Source: CAD feature listing. Evaluate the final solid. Frame: model axes, mm. Face numbers are marked on the shaded views. A direction names the side the tool comes from. Round coordinates to 2 decimals unless told otherwise and drop trailing zeros. Order: outer loops, then holes, each group sorted by start corner. A loop starts at its lowest first (then second) coordinate and runs counter-clockwise, first axis right, second up. Notation, with made-up numbers: M 73,-24 L 124,-24 A24 cw 124,9 Z; hole C -9.5,15.25 d11. An arc over 180 degrees is marked long. Use one line per item in the form item = value. Start each with the question number.
Q1. Reachability of the marked faces 1, 2, 3 and 4 from +Z, -Z, +X, -X, +Y, -Y: full face, straight path, thin tool, end or side. Return the list, or none.
Q2. Section C-C (y = -5). Return the cut outline in (x, z).
Q3. Section B-B (x = -6). Return the cut outline in (y, z), plus the area to 3 significant figures.
Q4. Pull-direction query (X, two-part tool) for the marked faces 5, 6, 7 and 8; classes: pulls with the +X half, pulls with the -X half, needs draft (parallel to the pull), parting line crosses it, or undercut.
Q5. Section D-D (y = -11). Return the cut outline in (x, z).
Q6. Section A-A (z = 4). Return the cut outline in (x, y), plus the area to 3 significant figures.
Q7. Material intervals for probe 1 along Z at (x, y) = (4, -3); probe 2 along Y at (x, z) = (-6, -2); probe 3 along X at (y, z) = (-1.25, 5.25), sorted ascending.
Q8. Contact query for flat-ended pins moving along their axis: pin 1 (2 mm diameter, centred on x = -2.5, y = -7.5, fed in from +Z); pin 2 (2 mm diameter, centred on x = 1, y = -2.5, fed in from -Z); pin 3 (3 mm diameter, centred on x = 8.5, y = -2.5, fed in from +Z); pin 4 (2.5 mm diameter, centred on x = -6, z = 4, fed in from -Y). Output: stop coordinate, or through.
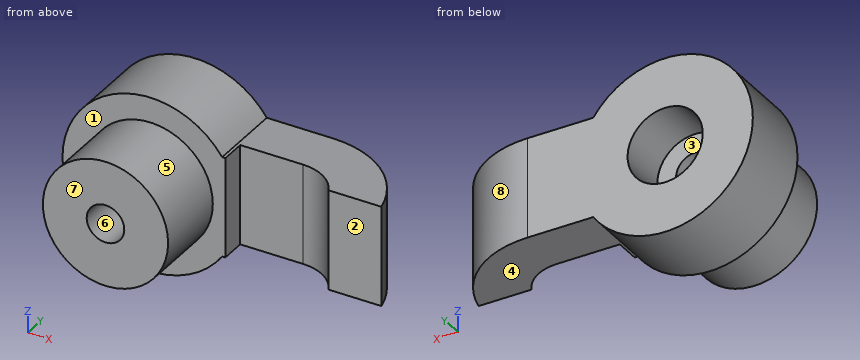
from build123d import *

# Parameters (mm, degrees)
EXTRUDE_1_DEPTH           = 8
EXTRUDE_2_DEPTH           = 6
SKETCH_5_R                = 5
EXTRUDE_3_DEPTH           = 6
HOLE_WIZARD_1_D           = 3
HOLE_WIZARD_1_DEPTH       = 30
HOLE_WIZARD_1_CBORE_D     = 6
HOLE_WIZARD_1_CBORE_DEPTH = 4


with BuildPart() as part:
    # 草图3 → 凸台-拉伸1 (new body)
    with BuildSketch(Plane.XY):
        with BuildLine():
            Line((0, 0), (5, 0))
            ThreePointArc((5, 0), (9.784396345, -1.68635165), (12.453978369, -6))
            Line((12.453978369, -6), (8.243547108, -6))
            ThreePointArc((8.243547108, -6), (6.905295111, -4.540192237), (5, -4))
            Line((5, -4), (0, -4))
            Line((0, -4), (0, 0))
        make_face()
    extrude(amount=EXTRUDE_1_DEPTH)

    # 草图4 → 凸台-拉伸2 (add)
    with BuildSketch(Plane(origin=(0, 0, 0), x_dir=(1, 0, 0), z_dir=(0, 1, 0))):
        with BuildLine():
            Line((-0.255437353, 0), (0, 0))
            Line((0, 0), (0, -8))
            Line((0, -8), (-0.255437353, -8))
            ThreePointArc((-0.255437353, -8), (-13, -4), (-0.255437353, 0))
        make_face()
    extrude(amount=-EXTRUDE_2_DEPTH)

    # 草图5 → 凸台-拉伸3 (add)
    with BuildSketch(Plane.XZ.offset(6)):
        with Locations((-6, 4)):
            Circle(SKETCH_5_R)
    extrude(amount=EXTRUDE_3_DEPTH)

    # 孔1
    with Locations(Plane(origin=(-6, 0, 4), x_dir=(0, 0, 1), z_dir=(0, 1, 0))):
        with Locations((0, 0)):
            CounterBoreHole(HOLE_WIZARD_1_D / 2, HOLE_WIZARD_1_CBORE_D / 2, HOLE_WIZARD_1_CBORE_DEPTH, depth=HOLE_WIZARD_1_DEPTH)


solid = part.part
Results list:
q1.face_1 = -Y
q1.face_2 = +Z, -Z, +X, -Y
q1.face_3 = +Y
q1.face_4 = -Z, +X, +Y, -Y
q2.outline = M -0.26,0 L 0,0 L 0,8 L -0.26,8 A7 ccw long Z; M 7.5,0 L 12.16,0 L 12.16,8 L 7.5,8 Z; hole C -6,4 d3
q3.outline = M -12,-1 L -6,-1 L -6,-3 L 0,-3 L 0,1 L -4,1 L -4,2.5 L -12,2.5 Z; M -12,5.5 L -4,5.5 L -4,7 L 0,7 L 0,11 L -6,11 L -6,9 L -12,9 Z
q3.area = 96.0 mm2
q4.face_5 = parting line crosses it
q4.face_6 = undercut
q4.face_7 = needs draft
q4.face_8 = pulls with the +X half
q5.outline = C -6,4 d10; hole C -6,4 d3
q6.outline = M -13,-6 L -11,-6 L -11,-12 L -7.5,-12 L -7.5,-4 L -9,-4 L -9,0 L -13,0 Z; M -4.5,-12 L -1,-12 L -1,-6 L 0,-6 L 0,-4 L 5,-4 A3.63 cw 8.24,-6 L 12.45,-6 A7.63 ccw 5,0 L -3,0 L -3,-4 L -4.5,-4 Z
q6.area = 139 mm2
q7.probe_1 = 0 to 8
q7.probe_2 = -6 to 0
q7.probe_3 = -12.89 to -8.73, -3.27 to 9.18
q8.pin_1 = 8.33
q8.pin_2 = 0
q8.pin_3 = 8
q8.pin_4 = through
